Can you work these out from the model? Positions are in its coordinate system, mm. Face numbers are marked on the shaded views. A direction names the side the tool comes from. Coordinates: 2 decimals unless noted, no trailing zeros. Order: outer loops, then holes, each group sorted by start corner. A loop starts at its lowest first (then second) coordinate and runs counter-clockwise, first axis right, second up. Notation, with made-up numbers: (22.5, 78.5) -> (55.5, 78.5) arc R31 ccw to (55.5, 117.5) -> close; hole circle Ø8 at (-28, -18.75). An arc over 180 degrees is marked (long way). Answer in a Markdown table with one row per item.
```python
from build123d import *

# Parameters (mm, degrees)
BOSS_EXTRUDE1_DEPTH = 52
BOSS_EXTRUDE2_START = -22
BOSS_EXTRUDE2_DEPTH = 8


with BuildPart() as part:
    # Sketch1 → Boss-Extrude1 (new body)
    with BuildSketch(Plane.XY):
        with BuildLine():
            Line((-4.5, 20.444512863), (-4.5, 3))
            Line((-4.5, 3), (0, 3))
            Line((0, 3), (4.5, 3))
            Line((4.5, 3), (4.5, 20.444512863))
            ThreePointArc((4.5, 20.444512863), (17.783419244, 28.414047854), (23, 43))
            Line((23, 43), (15, 43))
            ThreePointArc((15, 43), (0, 28), (-15, 43))
            Line((-15, 43), (-23, 43))
            ThreePointArc((-23, 43), (-17.783419244, 28.414047854), (-4.5, 20.444512863))
        make_face()
        Polygon((-4.5, 3), (-37.5, 3), (-37.5, -3), (37.5, -3), (37.5, 3), (4.5, 3), (0, 3), align=None)
    extrude(amount=-BOSS_EXTRUDE1_DEPTH)

    # Sketch7 → Boss-Extrude2 (add)
    with BuildSketch(Plane.XY.offset(BOSS_EXTRUDE2_START)):
        with BuildLine():
            Line((23, 43), (37.5, 3))
            Line((37.5, 3), (4.5, 3))
            Line((4.5, 3), (4.5, 20.444512863))
            ThreePointArc((4.5, 20.444512863), (17.783419244, 28.414047854), (23, 43))
        make_face()
    extrude(amount=-BOSS_EXTRUDE2_DEPTH)


solid = part.part
```
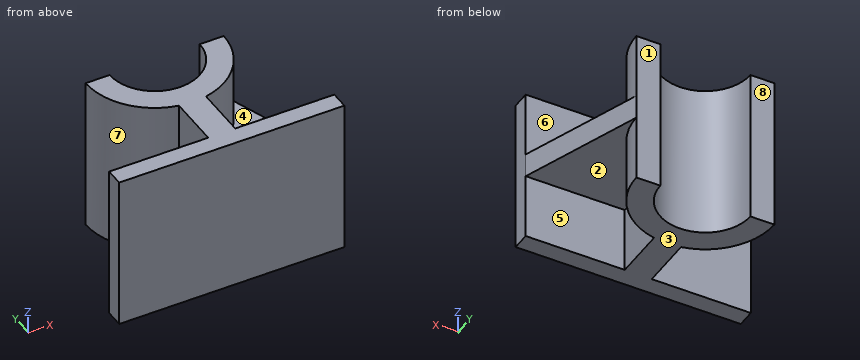
(1) Suppose I cut it at C-C (x = -21). Please give me the cut outline in (y, z), and give its area (3 significant figures).
Response values:
| item | result |
|---|---|
| outline | (-3, -52) -> (3, -52) -> (3, 0) -> (-3, 0) -> close; (33.62, -52) -> (43, -52) -> (43, 0) -> (33.62, 0) -> close |
| area | 800 mm2 |
(2) I need wall thicknesses on line 1 (Y direction, x = -32.5, z = -24); line 2 (X direction, y = 38, z = -35); line 3 (Z direction, x = 17, y = 18.5). Which ranges of each line are inside material? Lowest first, please. Write a range as [from, to].
Response values:
| item | result |
|---|---|
| line 1 | [-3, 3] |
| line 2 | [-22.45, -14.14], [14.14, 22.45] |
| line 3 | [-30, -22] |
(3) Will these pins go through, and if not, where does the flat tip stop? pin 1 Ø5 at (y, z) = (9, -14.5) entering from -X; pin 2 Ø10 at (x, y) = (2.5, 14.5) entering from +Z; pin 3 Ø1.5 at (y, z) = (29.5, -41) entering from -X; pin 4 Ø12 at (y, z) = (35.5, -16.5) entering from -X.
Response values:
| item | result |
|---|---|
| pin 1 | x = -4.5 |
| pin 2 | z = 0 |
| pin 3 | x = -19.14 |
| pin 4 | x = -22.95 |
(4) Suppose I cut it at D-D (x = 0). Please give me the cut outline in (y, z), and give its area (3 significant figures).
Response values:
| item | result |
|---|---|
| outline | (-3, -52) -> (28, -52) -> (28, 0) -> (-3, 0) -> close |
| area | 1,610 mm2 |
(5) Suppose I cut it at B-B (z = -41). Please give me the cut outline in (x, y).
Response values:
| item | result |
|---|---|
| outline | (-37.5, -3) -> (37.5, -3) -> (37.5, 3) -> (4.5, 3) -> (4.5, 20.44) arc R23 ccw to (23, 43) -> (15, 43) arc R15 cw to (-15, 43) -> (-23, 43) arc R23 ccw to (-4.5, 20.44) -> (-4.5, 3) -> (-37.5, 3) -> close |
(6) We'd pull the mould along Y, two halves only. Please class the marked faces 1, 2, 3 and 4: +Y half, -Y half, draft (parallel to the pull), parting line (faces both ways), or undercut.
Response values:
| item | result |
|---|---|
| face 1 | +Y half |
| face 2 | undercut |
| face 3 | draft |
| face 4 | undercut |
(7) On a 3-axis mill with a long thin cutter (end or side, diameter ignored), from which of +Z, -Z, +X, -X, +Y, -Y can I reach the whole of each face in a straight line? I mean the marked faces 5, 6, 7 and 8. Say none if no direction works.
Response values:
| item | result |
|---|---|
| face 5 | -Z, +X |
| face 6 | +Z, +X |
| face 7 | +Z, -Z, -X |
| face 8 | +Z, -Z, +X, -X, +Y |
(8) Suppose I cut it at A-A (y = 32.5). Please give me the cut outline in (x, z), and give its area (3 significant figures).
Response values:
| item | result |
|---|---|
| outline | (-20.46, -52) -> (-10.71, -52) -> (-10.71, 0) -> (-20.46, 0) -> close; (10.71, -52) -> (20.46, -52) -> (20.46, -30) -> (26.81, -30) -> (26.81, -22) -> (20.46, -22) -> (20.46, 0) -> (10.71, 0) -> close |
| area | 1,060 mm2 |
